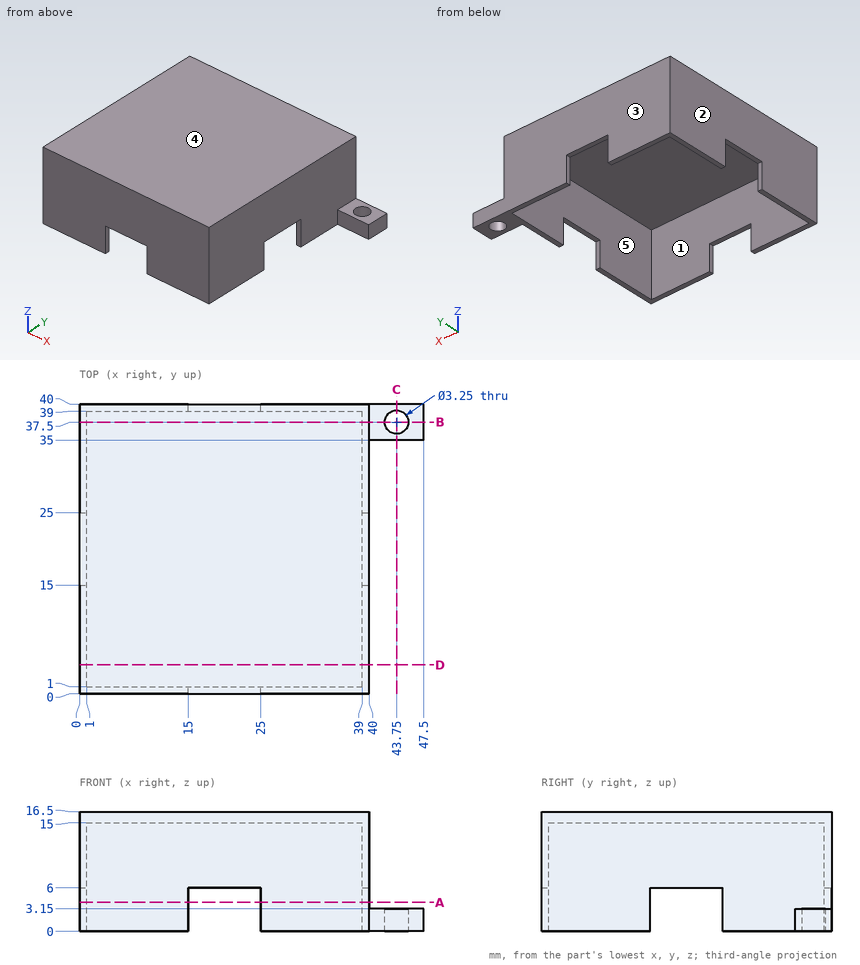
Geometry check sheet. Reference: drawing and pictorial views, mm from the part's lowest x, y, z. A direction names the side the tool comes from. Round coordinates to 2 decimals unless told otherwise and drop trailing zeros. Order: outer loops, then holes, each group sorted by start corner. A loop starts at its lowest first (then second) coordinate and runs counter-clockwise, first axis right, second up. Notation, with made-up numbers: (87, 61.5) - (111, 61.5) arc R22 ccw to (111, 79.5) - close; hole circle Ø6 at (74, 85). An arc over 180 degrees is marked (long way). Use a Markdown table: item, result. Add a question column.
1) Section check A-A (z = 4). Record the cut outline in (x, y).
2) Section check D-D (y = 4). Record the cut outline in (x, z).
3) Gauge pin test, flat ends, axial feed: P1, Ø1.1, axis at x = 0.5, y = 19, coming from the -Z side; P2, Ø2, axis at x = 19.5, y = 20.5, coming from the -Z side; P3, Ø1.5, axis at y = 12, z = 4, coming from the +X side. Record the tip position at first contact, or that the pin passes through.
4) Section check B-B (y = 37.5). Record the cut outline in (x, z) (3 decimals), then the cut area to 3 significant figures.
5) Thickness scan on line 1 along X through (y, z) = (13.5, 3); line 2 along Y through (x, z) = (43.75, 1.8) (3 decimals). Record the ranges inside material, lowest first.
6) Section check C-C (x = 43.75). Record the cut outline in (y, z) (3 decimals).
7) Mould release check, pull along X, two halves, no side actions. Record for the marked faces 1, 2 and 3: released by +X, released by -X, zero draft, split by the parting line, or undercut.
8) Set-up check for the marked faces 4 and 5: record each of +Z, -Z, +X, -X, +Y, -Y from which the full face is reachable in a straight line by a thin tool's end or side.
Established:
| question | item | result |
|---|---|---|
| 1 | outline | (0, 0) - (15, 0) - (15, 1) - (1, 1) - (1, 15) - (0, 15) - close; (0, 25) - (1, 25) - (1, 39) - (15, 39) - (15, 40) - (0, 40) - close; (25, 0) - (40, 0) - (40, 15) - (39, 15) - (39, 1) - (25, 1) - close; (25, 39) - (39, 39) - (39, 25) - (40, 25) - (40, 40) - (25, 40) - close |
| 2 | outline | (0, 0) - (1, 0) - (1, 15) - (39, 15) - (39, 0) - (40, 0) - (40, 16.5) - (0, 16.5) - close |
| 3 | P1 | z = 6 |
| 3 | P2 | z = 15 |
| 3 | P3 | x = 40 |
| 4 | outline | (0, 0) - (1, 0) - (1, 15) - (39, 15) - (39, 0) - (42.125, 0) - (42.125, 3.15) - (40, 3.15) - (40, 16.5) - (0, 16.5) - close; (45.375, 0) - (47.5, 0) - (47.5, 3.15) - (45.375, 3.15) - close |
| 4 | area | 103 mm2 |
| 5 | line 1 | 0 to 1, 39 to 40 |
| 5 | line 2 | 35 to 35.875, 39.125 to 40 |
| 6 | outline | (35, 0) - (35.875, 0) - (35.875, 3.15) - (35, 3.15) - close; (39.125, 0) - (40, 0) - (40, 3.15) - (39.125, 3.15) - close |
| 7 | face 1 | undercut |
| 7 | face 2 | released by -X |
| 7 | face 3 | zero draft |
| 8 | face 4 | +Z, +X, -X, +Y, -Y |
| 8 | face 5 | -Z |
